Could you check a few things on this model? Use its own coordinates, in mm. A direction names the side the tool comes from. Coordinates: 2 decimals unless noted, no trailing zeros. Order: outer loops, then holes, each group sorted by start corner. A loop starts at its lowest first (then second) coordinate and runs counter-clockwise, first axis right, second up. Notation, with made-up numbers: (-4, -26) - (16, -26) arc R9 cw to (16, -12) - close; hole circle Ø11 at (14, -14.5). An arc over 180 degrees is marked (long way). Answer as CSV lines item,"result". Start each with the question number.
1. For pin 1 (6 mm diameter, centred on y = 59.5, z = 145.5, fed in from +X); pin 2 (12.5 mm diameter, centred on x = -43.5, z = 743.5, fed in from -Y); pin 3 (12.5 mm diameter, centred on y = -53.5, z = 741.5, fed in from -X), each with a flat end and sliding along its axis, tell me the tip position at first contact or that it passes through.
2. I need wall thicknesses on probe 1 along Y at (x, z) = (127, 739); probe 2 along Y at (x, z) = (-150, 12); probe 3 along Z at (x, y) = (-128, -92). Which ranges of each line are inside material? Lowest first, please.
3. I want a section at C-C, the plane y = -31.5. List the corners of the cut face in (x, z) for me, and give its area (4 significant figures).
4. I want a section at A-A, the plane x = 127. List the corners of the cut face in (y, z) for me.
5. For faces 4 (the face through (-162, -159, 12)), 5 (the face through (131.268, -139.206, 737.325)), 6 (the face through (-2, 150, 737)), 7 (the face through (-1, 75, 370)), 8 (the face through (-3, 92, 25)), which set-ups out of +Z, -Z, +X, -X, +Y, -Y let a thin tool reach every point of the face, with its end or its side?
6. I want a section at B-B, the plane y = -114. List the corners of the cut face in (x, z) for me.
7. Thinking about a two-plate mould opening in X: for faces 1 (the face through (-122.732, 122.794, 737.325)), 2 (the face through (-75, -1, 370)), 3 (the face through (-2, -150, 737)), which applies, released by +X, released by -X, zero draft, split by the parting line, or undercut?
from build123d import *

# Parameters (mm, degrees)
F0_W     = 400
F0_H     = 400
F0_R     = 15
F1_DEPTH = 25
F2_W     = 150
F2_H     = 150
F3_DEPTH = 700
F4_W     = 300
F4_H     = 300
F4_R     = 9.25
F5_DEPTH = 25


with BuildPart() as f1:
    # F0 (on Top) → F1 (new body)
    with BuildSketch(Plane.XY):
        Rectangle(F0_W, F0_H)
        with Locations((-150, -150)):
            Circle(F0_R, mode=Mode.SUBTRACT)
        with Locations((150, -150)):
            Circle(F0_R, mode=Mode.SUBTRACT)
        with Locations((-150, 150)):
            Circle(F0_R, mode=Mode.SUBTRACT)
        with Locations((150, 150)):
            Circle(F0_R, mode=Mode.SUBTRACT)
    extrude(amount=F1_DEPTH)

    # F2 (on face) → F3 (join)
    with BuildSketch(Plane.XY.offset(25)):
        Rectangle(F2_W, F2_H)
    extrude(amount=F3_DEPTH)

    # F4 (on face) → F5 (join)
    with BuildSketch(Plane.XY.offset(725)):
        Rectangle(F4_W, F4_H)
        with Locations((-127, -131)):
            Circle(F4_R, mode=Mode.SUBTRACT)
        with Locations((127, -131)):
            Circle(F4_R, mode=Mode.SUBTRACT)
        with Locations((-127, 131)):
            Circle(F4_R, mode=Mode.SUBTRACT)
        with Locations((127, 131)):
            Circle(F4_R, mode=Mode.SUBTRACT)
    extrude(amount=F5_DEPTH)


solid = f1.part
Solved:
1,pin 1,"stops at x = 75"
1,pin 2,"stops at y = -150"
1,pin 3,"stops at x = -150"
2,probe 1,"y = -150 to -140.25, -121.75 to 121.75, 140.25 to 150"
2,probe 2,"y = -200 to -165, -135 to 135, 165 to 200"
2,probe 3,"z = 0 to 25, 725 to 750"
3,outline,"(-200, 0) - (200, 0) - (200, 25) - (75, 25) - (75, 725) - (150, 725) - (150, 750) - (-150, 750) - (-150, 725) - (-75, 725) - (-75, 25) - (-200, 25) - close"
3,area,"122,500 mm2"
4,outline,"(-200, 0) - (200, 0) - (200, 25) - (-200, 25) - close; (-150, 725) - (-140.25, 725) - (-140.25, 750) - (-150, 750) - close; (-121.75, 725) - (121.75, 725) - (121.75, 750) - (-121.75, 750) - close; (140.25, 725) - (150, 725) - (150, 750) - (140.25, 750) - close"
5,face 4,"-Z"
5,face 5,"+Z"
5,face 6,"+Z, +X, -X, +Y"
5,face 7,"+X, -X, +Y"
5,face 8,"none"
6,outline,"(-200, 0) - (200, 0) - (200, 25) - (-200, 25) - close; (-150, 725) - (150, 725) - (150, 750) - (-150, 750) - close"
7,face 1,"undercut"
7,face 2,"released by -X"
7,face 3,"zero draft"
